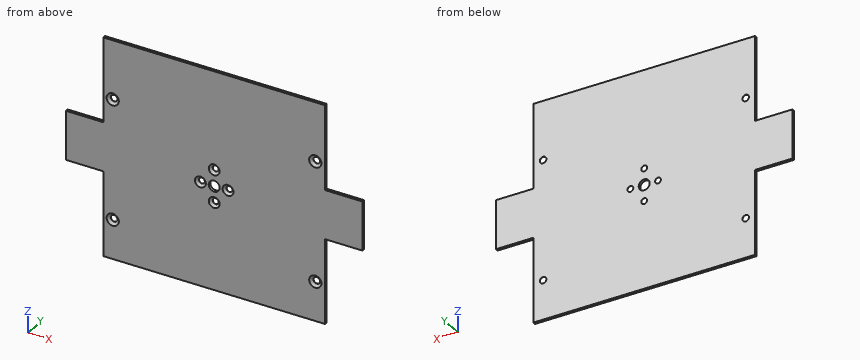
```python
from build123d import *

# Parameters (mm, degrees)
BOSS_EXTRUDE1_DEPTH                            = 1.5875
CSK_FOR_6_FLAT_HEAD_MACHINE_SCREW_2_COUNT      = 2
CSK_FOR_6_FLAT_HEAD_MACHINE_SCREW_2_PITCH      = 69.85
CSK_FOR_6_FLAT_HEAD_MACHINE_SCREW_3_COUNT      = 2
CSK_FOR_6_FLAT_HEAD_MACHINE_SCREW_3_PITCH      = 136.672594638
CSK_FOR_6_FLAT_HEAD_MACHINE_SCREW_4_COUNT      = 2
CSK_FOR_6_FLAT_HEAD_MACHINE_SCREW_4_PITCH      = 117.475
SKETCH4_R                                      = 3.175
CUT_EXTRUDE1_DEPTH                             = 107.878457248
CSK_FOR_M3_FLAT_HEAD_MACHINE_SCREW2_AT_2_COUNT = 2
CSK_FOR_M3_FLAT_HEAD_MACHINE_SCREW2_AT_2_PITCH = 16
CSK_FOR_M3_FLAT_HEAD_MACHINE_SCREW2_AT_3_COUNT = 2
CSK_FOR_M3_FLAT_HEAD_MACHINE_SCREW2_AT_3_PITCH = 12.419742348
CSK_FOR_M3_FLAT_HEAD_MACHINE_SCREW2_AT_4_COUNT = 2
CSK_FOR_M3_FLAT_HEAD_MACHINE_SCREW2_AT_4_PITCH = 12.419742348


with BuildPart() as part:
    # Sketch1 → Boss-Extrude1 (new body)
    with BuildSketch(Plane(origin=(0, 0, 0), x_dir=(1, 0, 0), z_dir=(0, 1, 0))):
        Polygon((-64.29375, 63.53175), (64.29375, 63.53175), (64.29375, 14.25575), (85.931375, 14.25575), (85.931375, -14.25575), (64.29375, -14.25575), (64.29375, -63.53175), (-64.29375, -63.53175), (-64.29375, -14.25575), (-85.931375, -14.25575), (-85.931375, 14.25575), (-64.29375, 14.25575), align=None)
    extrude(amount=BOSS_EXTRUDE1_DEPTH)

    # Sketch2 → CSK for #6 Flat Head Machine Screw (100)1 (revolve, cut)
    with BuildSketch(Plane(origin=(-58.848625, 0, 29.17825), x_dir=(0, 0, -1), z_dir=(1, 0, 0))):
        Polygon((0, 0), (0, 1.5875), (1.89865, 1.5875), (1.89865, 1.380025208), (3.5433, 0), align=None)
    csk_for_6_flat_head_machine_screw_100 = revolve(axis=Axis((-58.848625, -6.35, 29.17825), (0, 1, 0)), mode=Mode.SUBTRACT)

    # CSK for _6 Flat Head Machine Screw _ 2: CSK for #6 Flat Head Machine Screw (100)1 ×2
    with Locations(*[(0, 0, -i * CSK_FOR_6_FLAT_HEAD_MACHINE_SCREW_2_PITCH) for i in range(1, CSK_FOR_6_FLAT_HEAD_MACHINE_SCREW_2_COUNT)]):
        add(csk_for_6_flat_head_machine_screw_100, mode=Mode.SUBTRACT)

    # CSK for _6 Flat Head Machine Screw _ 3: CSK for #6 Flat Head Machine Screw (100)1 ×2
    with Locations(*[Vector(0.8595358880206613, 0, -0.5110753928771502) * (i * CSK_FOR_6_FLAT_HEAD_MACHINE_SCREW_3_PITCH) for i in range(1, CSK_FOR_6_FLAT_HEAD_MACHINE_SCREW_3_COUNT)]):
        add(csk_for_6_flat_head_machine_screw_100, mode=Mode.SUBTRACT)

    # CSK for _6 Flat Head Machine Screw _ 4: CSK for #6 Flat Head Machine Screw (100)1 ×2
    with Locations(*[(i * CSK_FOR_6_FLAT_HEAD_MACHINE_SCREW_4_PITCH, 0, 0) for i in range(1, CSK_FOR_6_FLAT_HEAD_MACHINE_SCREW_4_COUNT)]):
        add(csk_for_6_flat_head_machine_screw_100, mode=Mode.SUBTRACT)

    # Sketch4 → Cut-Extrude1 (cut, through all)
    with BuildSketch(Plane.XZ):
        with Locations(Location((0, -3.175, 0), (0, 0, 270))):
            Circle(SKETCH4_R)
    extrude(amount=-CUT_EXTRUDE1_DEPTH, mode=Mode.SUBTRACT)

    # Sketch5 → CSK for M3 Flat Head Machine Screw2 (revolve, cut)
    with BuildSketch(Plane(origin=(8, 0, -3.175), x_dir=(0, 0, -1), z_dir=(1, 0, 0))):
        Polygon((0, 0), (0, 1.5875), (1.7, 1.5875), (1.7, 1.45), (3.15, 0), align=None)
    csk_for_m3_flat_head_machine_screw2 = revolve(axis=Axis((8, -6.35, -3.175), (0, 1, 0)), mode=Mode.SUBTRACT)

    # CSK for M3 Flat Head Machine Screw2 at 2: CSK for M3 Flat Head Machine Screw2 ×2
    with Locations(*[(-i * CSK_FOR_M3_FLAT_HEAD_MACHINE_SCREW2_AT_2_PITCH, 0, 0) for i in range(1, CSK_FOR_M3_FLAT_HEAD_MACHINE_SCREW2_AT_2_COUNT)]):
        add(csk_for_m3_flat_head_machine_screw2, mode=Mode.SUBTRACT)

    # CSK for M3 Flat Head Machine Screw2 at 3: CSK for M3 Flat Head Machine Screw2 ×2
    with Locations(*[Vector(-0.6441357457827798, 0, -0.7649111981170509) * (i * CSK_FOR_M3_FLAT_HEAD_MACHINE_SCREW2_AT_3_PITCH) for i in range(1, CSK_FOR_M3_FLAT_HEAD_MACHINE_SCREW2_AT_3_COUNT)]):
        add(csk_for_m3_flat_head_machine_screw2, mode=Mode.SUBTRACT)

    # CSK for M3 Flat Head Machine Screw2 at 4: CSK for M3 Flat Head Machine Screw2 ×2
    with Locations(*[Vector(-0.6441357457827798, 0, 0.7649111981170509) * (i * CSK_FOR_M3_FLAT_HEAD_MACHINE_SCREW2_AT_4_PITCH) for i in range(1, CSK_FOR_M3_FLAT_HEAD_MACHINE_SCREW2_AT_4_COUNT)]):
        add(csk_for_m3_flat_head_machine_screw2, mode=Mode.SUBTRACT)


solid = part.part
```
Could you check a few things on this model? Use its own coordinates, in mm. Give positions to 0.01 mm unless a question says otherwise; leave off trailing zeros. Order: outer loops, then holes, each group sorted by start corner. A loop starts at its lowest first (then second) coordinate and runs counter-clockwise, first axis right, second up.
Q1. I'm going to push flat-ended pins straight in: P1, Ø4.5, axis at x = -8, z = -3.175, coming from the -Y side; P2, Ø2, axis at x = 0, z = -12.675, coming from the +Y side; P3, Ø4.5, axis at x = 58.63, z = -40.67, coming from the +Y side; P4, Ø0.5, axis at y = 1, z = 35.5, coming from the +X side. Where does each tip first touch, or does it pass through?
Q2. If I drill on line 1 along Z through (x, y) = (2, 0.45); line 2 along X through (y, z) = (0.1, -1); line 3 along X through (y, z) = (0.25, -48.5), over which ranges is the centre line in solid material (lowest first)?
Q3. Suppose I cut it at A-A, the plane y = 0.8. Count the separate pieces of the cut face and the enclosed holes in it, and give its area (3 significant figures).
Q4. Suppose I cut it at B-B, the plane x = -75. Write out the boundary of the cut face in (y, z), and give its area (3 significant figures).
Q5. Suppose I cut it at C-C, the plane z = -22. Write out the boundary of the cut face in (x, y), and give its area (3 significant figures).
Solution:
1. P1: stops at y = 0.9
1. P2: passes through
1. P3: stops at y = 1.59
1. P4: stops at x = 64.29
2. line 1: z = -63.53 to -14.49, -10.86 to -5.64, -0.71 to 4.51, 8.14 to 63.53
2. line 2: x = -85.93 to -10.14, -5.86 to -2.31, 2.31 to 5.86, 10.14 to 85.93
2. line 3: x = -64.29 to 64.29
3. separate pieces: 1
3. enclosed holes: 9
3. area: 17,400 mm2
4. outline: (0, -14.26) - (1.59, -14.26) - (1.59, 14.26) - (0, 14.26) - close
4. area: 45.3 mm2
5. outline: (-64.29, 0) - (64.29, 0) - (64.29, 1.59) - (-64.29, 1.59) - close
5. area: 204 mm2
